Read the model definition and answer for the solid it produces. Units are mm, in the model's axes. Face numbers are marked on the shaded views. A direction names the side the tool comes from. Round coordinates to 2 decimals unless told otherwise and drop trailing zeros. Write each loop counter-clockwise with the first axis right and the second up, starting at its lowest first coordinate (ties: lowest second). Pieces come first, ordered by that corner, then holes. Notation, with made-up numbers: (13, -25.75) - (19, -25.75) arc R19 cw to (19, -1.75) - close; hole circle Ø1 at (58.5, 73.5). An arc over 180 degrees is marked (long way). Use one line per item in the form item = value. Start each with the question number.
1) Consider line 1 along Y through (x, z) = (-32, 0); line 2 along X through (y, z) = (98.5, 9); line 3 along X through (y, z) = (73.5, 22). Determine where each line is inside the solid, lowest interval first. Write a range as from..to.
2) For the marked faces 1, 2, 3, 4 and 5, determine the directions among +Z, -Z, +X, -X, +Y, -Y from which every point of the face is accessible in a straight line to the end or side of a thin tool.
3) For a pull along X with two mould halves and no side action, classify the marked faces 6, 7 and 8 as released by +X, released by -X, zero draft, split by the parting line, or undercut.
4) Each of these flat-tipped pins is pushed along its axis until it touches: pin 1 (4.5 mm diameter, centred on y = 123.5, z = -18, fed in from +X); pin 2 (1 mm diameter, centred on x = 68.5, z = -14.5, fed in from +Y); pin 3 (15 mm diameter, centred on y = 70, z = 0, fed in from +X). Where does it stop, or does it pass through?
5) The part is cut by section A-A, the plane y = 43.5. Give the vertices of the cut face in (x, z), plus the area to 3 significant figures.
6) The part is cut by section B-B, the plane z = 0. Give the vertices of the cut face in (x, y).
7) The part is cut by section C-C, the plane y = 70. Give the vertices of the cut face in (x, z), plus the area to 3 significant figures.
8) The part is cut by section D-D, the plane z = -15. Give the vertices of the cut face in (x, y).
from build123d import *

# Parameters (mm, degrees)
BOSS_EXTRUDE1_DEPTH = 37.5
SKETCH2_R           = 12.5
CUT_EXTRUDE1_DEPTH  = 100


with BuildPart() as part:
    # Sketch1 → Boss-Extrude1 (new body, symmetric)
    with BuildSketch(Plane.XY):
        Polygon((-95, 39.909181495), (-35, 39.909181495), (-35, 120), (-45, 120), (-45, 90), (-55.365508708, 121.312096701), (-55.365508708, 130), (-25, 130), (-25, 30), (40, 10), (105, 30), (105, 0), (-105, 0), (-105, 130), (-75.365508708, 130), (-75.365508708, 121.312096701), (-85, 90), (-85, 120), (-95, 120), align=None)
    extrude(amount=BOSS_EXTRUDE1_DEPTH, both=True)

    # Sketch2 → Cut-Extrude1 (cut)
    with BuildSketch(Plane.ZY.offset(105)):
        with Locations((0, 70)):
            Circle(SKETCH2_R)
    extrude(amount=-CUT_EXTRUDE1_DEPTH, mode=Mode.SUBTRACT)


solid = part.part
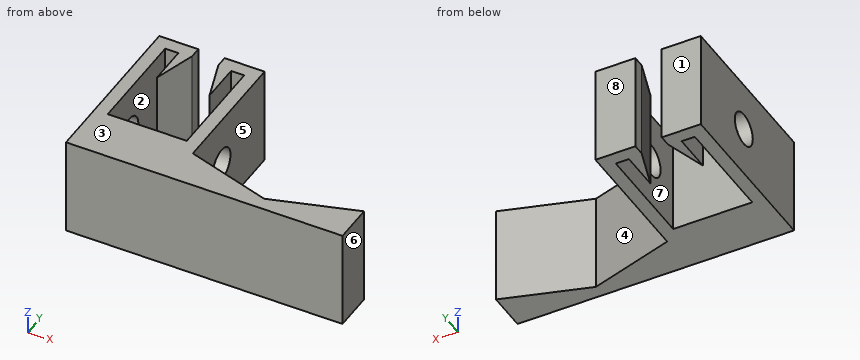
Geometry results:
q1.line_1 = 0..57.5, 82.5..130
q1.line_2 = -105..-95, -85..-82.38, -47.81..-45, -35..-25
q1.line_3 = -105..-95, -35..-25
q2.face_1 = +Z, -Z, +X, -X, +Y
q2.face_2 = +Z, -Z
q2.face_3 = +Z, +X, -X, +Y, -Y
q2.face_4 = +Z, -Z, +Y
q2.face_5 = +Z, -Z, +X, +Y
q3.face_6 = released by +X
q3.face_7 = undercut
q3.face_8 = zero draft
q4.pin_1 = -25
q4.pin_2 = 18.92
q4.pin_3 = through
q5.outline = (-105, -37.5) - (-95, -37.5) - (-95, 37.5) - (-105, 37.5) - close; (-35, -37.5) - (-25, -37.5) - (-25, 37.5) - (-35, 37.5) - close
q5.area = 1,500 mm2
q6.outline = (-105, 0) - (105, 0) - (105, 30) - (40, 10) - (-25, 30) - (-25, 57.5) - (-35, 57.5) - (-35, 39.91) - (-95, 39.91) - (-95, 57.5) - (-105, 57.5) - close; (-105, 82.5) - (-95, 82.5) - (-95, 120) - (-85, 120) - (-85, 90) - (-75.37, 121.31) - (-75.37, 130) - (-105, 130) - close; (-55.37, 121.31) - (-45, 90) - (-45, 120) - (-35, 120) - (-35, 82.5) - (-25, 82.5) - (-25, 130) - (-55.37, 130) - close
q7.outline = (-105, -37.5) - (-95, -37.5) - (-95, -12.5) - (-105, -12.5) - close; (-105, 12.5) - (-95, 12.5) - (-95, 37.5) - (-105, 37.5) - close; (-35, -37.5) - (-25, -37.5) - (-25, -12.5) - (-35, -12.5) - close; (-35, 12.5) - (-25, 12.5) - (-25, 37.5) - (-35, 37.5) - close
q7.area = 1,000 mm2
q8.outline = (-105, 0) - (105, 0) - (105, 30) - (40, 10) - (-25, 30) - (-25, 130) - (-55.37, 130) - (-55.37, 121.31) - (-45, 90) - (-45, 120) - (-35, 120) - (-35, 39.91) - (-95, 39.91) - (-95, 120) - (-85, 120) - (-85, 90) - (-75.37, 121.31) - (-75.37, 130) - (-105, 130) - close
